```python
from build123d import *

# Parameters (mm, degrees)
BOSS_EXTRUDE1_START = -1.675
SKETCH2_R           = 0.5
BOSS_EXTRUDE1_DEPTH = 1.675
CIRPATTERN1_COUNT   = 2


with BuildPart() as part:
    # Sketch1 → Revolve1 (revolve)
    with BuildSketch(Plane.XY, mode=Mode.PRIVATE) as revolve1_sk:
        Polygon((2.25, 0), (1.25, 0), (1.25, 0.76), (2, 0.76), (2, 1.69), (3.5, 1.69), (3.5, -2.21), (2.25, -2.21), align=None)
    revolve(revolve1_sk.sketch.rotate(Axis((0, 0, 0), (0, -1, 0)), 180), axis=Axis((0, 0, 0), (0, -1, 0)))

    # Sketch2 → Boss-Extrude1 (add)
    with BuildSketch(Plane(origin=(0, 1.69, 0), x_dir=(1, 0, 0), z_dir=(0, 1, 0)).offset(BOSS_EXTRUDE1_START)):
        with BuildLine():
            Line((-1.905, 6.5278), (-1.905, 2.93614969))
            ThreePointArc((-1.905, 2.93614969), (0, 3.5), (1.905, 2.93614969))
            Line((1.905, 2.93614969), (1.905, 6.5278))
            ThreePointArc((1.905, 6.5278), (0, 8.4328), (-1.905, 6.5278))
        make_face()
        with Locations(Location((0, 6.5278, 0), (0, 0, 180))):
            Circle(SKETCH2_R, mode=Mode.SUBTRACT)
        with Locations(Location((0, 4.5278, 0), (0, 0, 180))):
            Circle(SKETCH2_R, mode=Mode.SUBTRACT)
    boss_extrude1 = extrude(amount=BOSS_EXTRUDE1_DEPTH)

    # CirPattern1: Boss-Extrude1 ×2 about axis
    cirpattern1_axis = Axis((0, 0, 0), (0, 1, 0))
    for i in range(1, CIRPATTERN1_COUNT):
        add(boss_extrude1.rotate(cirpattern1_axis, i * 360 / CIRPATTERN1_COUNT))


solid = part.part
```
Could you check a few things on this model? Use its own coordinates, in mm. A direction names the side the tool comes from. Round coordinates to 2 decimals unless told otherwise and drop trailing zeros. Loops run counter-clockwise (first coordinate to the right, second up) from the corner with the lowest first, then second, coordinate; pieces in that order, holes last. Notation, with made-up numbers: M 22.25,65.5 L 58.25,65.5 A9 ccw 58.25,77.5 Z; hole C 33.5,-21.5 d8. An arc over 180 degrees is marked long. Put each result on its own line as item: value.
Q1. Thinking about a two-plate mould opening in Z: for faces 4 (the face through (3.497, -0.721, -0.154)), 5 (the face through (-2.3, -2.21, 0.7)), 6 (the face through (-1, 0, 1)), 7 (the face through (-0.042, 0.841, 8.432)), which applies, released by +Z, released by -Z, zero draft, split by the parting line, or undercut?
Check result:
face 4: split by the parting line
face 5: zero draft
face 6: undercut
face 7: released by +Z
Q2. Imagine slicing it at A-A (z = 0). Write out the boundary of the cut face in (x, y), then the cut area to 3 significant figures.
Check result:
outline: M -3.5,-2.21 L -2.25,-2.21 L -2.25,0 L -1.25,0 L -1.25,0.76 L -2,0.76 L -2,1.69 L -3.5,1.69 Z; M 1.25,0 L 2.25,0 L 2.25,-2.21 L 3.5,-2.21 L 3.5,1.69 L 2,1.69 L 2,0.76 L 1.25,0.76 Z
area: 11.7 mm2
Q3. Imagine slicing it at B-B (x = 1). Write out the boundary of the cut face in (y, z) (3 decimals).
Check result:
outline: M -2.21,-3.354 L 0.015,-3.354 L 0.015,-8.149 L 1.69,-8.149 L 1.69,-1.732 L 0.76,-1.732 L 0.76,-0.75 L 0,-0.75 L 0,-2.016 L -2.21,-2.016 Z; M -2.21,2.016 L 0,2.016 L 0,0.75 L 0.76,0.75 L 0.76,1.732 L 1.69,1.732 L 1.69,8.149 L 0.015,8.149 L 0.015,3.354 L -2.21,3.354 Z
Q4. On a 3-axis mill with a long thin cutter (end or side, diameter ignored), from which of +Z, -Z, +X, -X, +Y, -Y can I reach the whole of each face in a straight line? I mean faces 1 (the face through (1.905, 1, -5)), 2 (the face through (0, 1, 2)), 3 (the face through (1.905, 1, 5)). Say none if no direction works.
Check result:
face 1: -Z, +X, +Y, -Y
face 2: +Y
face 3: +Z, +X, +Y, -Y
Q5. I need wall thicknesses on probe 1 along Z at (x, y) = (0, 0.2); probe 2 along Z at (x, y) = (0, 1.35); probe 3 along X at (y, z) = (1.3, 3) (3 decimals). Which ranges of each line are inside material? Lowest first, please.
Check result:
probe 1: -8.43 to -7.03, -6.03 to -5.03, -4.03 to -1.25, 1.25 to 4.03, 5.03 to 6.03, 7.03 to 8.43
probe 2: -8.43 to -7.03, -6.03 to -5.03, -4.03 to -2, 2 to 4.03, 5.03 to 6.03, 7.03 to 8.43
probe 3: -1.905 to 1.905
Q6. Imagine slicing it at C-C (y = 1.3). Write out the boundary of the cut face in (x, z) (3 decimals).
Check result:
outline: M -1.905,-6.528 A1.905 ccw 1.905,-6.528 L 1.905,-2.936 A3.5 ccw 1.905,2.936 L 1.905,6.528 A1.905 ccw -1.905,6.528 L -1.905,2.936 A3.5 ccw -1.905,-2.936 Z; hole C 0,0 d4; hole C 0,-6.528 d1; hole C 0,-4.528 d1; hole C 0,4.528 d1; hole C 0,6.528 d1
Q7. For pin 1 (1 mm diameter, centred on x = -0.5, y = -1, fed in from +Z); pin 2 (4 mm diameter, centred on x = -0.5, z = 5, fed in from -Y); pin 3 (1.5 mm diameter, centred on y = 1, z = 3.5, fed in from -X); pin 4 (1.5 mm diameter, centred on y = -1, z = 2.5, fed in from -X), each with a flat end and sliding along its axis, tell me the tip position at first contact or that it passes through.
Check result:
pin 1: z = 3.5
pin 2: y = -2.21
pin 3: x = -2.17
pin 4: x = -3.03
Q8. Imagine slicing it at D-D (x = 0). State how many separate pieces and enclosed holes the cut face has, then the cut area to 3 significant figures.
Check result:
separate pieces: 6
enclosed holes: 0
area: 21.6 mm2
